from build123d import *

# Parameters (mm, degrees)
SALIENTE_EXTRUIR1_DEPTH      = 20
SALIENTE_EXTRUIR1_DEPTH_BACK = 15
CROQUIS1_R                   = 3.25
CROQUIS1_3_R                 = 7.5
CROQUIS1_3_R_2               = 3.25
SALIENTE_EXTRUIR2_DEPTH      = 3
SALIENTE_EXTRUIR3_DEPTH      = 2


with BuildPart() as part:
    # Croquis1 → Saliente-Extruir1 (new, two sides: drawn at the far end of the back side and taken through both)
    with BuildSketch(Plane(origin=(0, 0, 0), x_dir=(1, 0, 0), z_dir=(0, 1, 0)).offset(-SALIENTE_EXTRUIR1_DEPTH_BACK)):
        with Locations(Location((0, 0, 0), (0, 0, 270))):
            Circle(CROQUIS1_R)
    extrude(amount=SALIENTE_EXTRUIR1_DEPTH + SALIENTE_EXTRUIR1_DEPTH_BACK)

    # Croquis1_3 → Saliente-Extruir2 (add, symmetric)
    with BuildSketch(Plane(origin=(0, 0, 0), x_dir=(1, 0, 0), z_dir=(0, 1, 0))):
        with Locations(Location((0, 0, 0), (0, 0, 270))):
            Circle(CROQUIS1_3_R)
        with Locations(Location((0, 0, 0), (0, 0, 270))):
            Circle(CROQUIS1_3_R_2, mode=Mode.SUBTRACT)
    extrude(amount=SALIENTE_EXTRUIR2_DEPTH, both=True)

    # Croquis2 → Saliente-Extruir3 (add)
    with BuildSketch(Plane(origin=(0, 20, 0), x_dir=(1, 0, 0), z_dir=(0, 1, 0))):
        with BuildLine():
            Line((0, 3.25), (20, 3.25))
            ThreePointArc((20, 3.25), (23.25, 0), (20, -3.25))
            Line((20, -3.25), (0, -3.25))
            ThreePointArc((0, -3.25), (-3.25, 0), (0, 3.25))
        make_face()
    extrude(amount=SALIENTE_EXTRUIR3_DEPTH)


solid = part.part
Design review of the part built by this model. Coordinates are the model's own, in mm. A direction names the side the tool comes from. Give positions to 0.01 mm unless a question says otherwise; leave off trailing zeros. Loops run counter-clockwise (first coordinate to the right, second up) from the corner with the lowest first, then second, coordinate; pieces in that order, holes last. Notation, with made-up numbers: (32.5, 80) - (58.5, 80) arc R24 cw to (58.5, 115) - close; hole circle Ø5 at (-10.5, 18.5). An arc over 180 degrees is marked (long way). Use CSV: the item, a comma, the result in double quotes. Start each with the question number.
1. Add section B-B (x = 5.5). State the section outline as (y, z) points.
2. Add section A-A (z = 0). State the section outline as (x, y) points.
3. Add section D-D (x = 19). State the section outline as (y, z) points.
4. Add section C-C (y = -12). State the section outline as (x, z) points.
5. Insertion check: P1, Ø0.6, axis at x = 12.5, y = 21, coming from the -Z side; P2, Ø5, axis at y = -1, z = -3, coming from the -X side; P3, Ø1.5, axis at x = -0.5, y = -8.5, coming from the +Z side. Each pin has a flat end and moves straight along its axis. Give the tip position at first contact, or say it passes through.
6. Wall thickness on L1, parallel to Y at x = -3, z = 3.25; L2, parallel to X at y = -13, z = 0; L3, parallel to Z at x = 21, y = 20.5: over which ranges is each line inside the solid? List them lowest first.
7. Machinability: for faces 4 (the flat face through (-2, 3, 3)), 5 (the flat face through (-2, -3, 3)), 6 (the flat face through (10, 21, -3.25)), 7 (the flat face through (10, 21, 3.25)), which of the approach directions +Z, -Z, +X, -X, +Y, -Y give a long, thin tool a straight path to every point of the face, cutting with its end or side? Answer none if there is none.
8. Draft analysis for pull direction Y (two halves, no side actions). For faces 1 (the flat face through (0, -15, 0)), 2 (the cylindrical face through (23.25, 20.99, -0.07)), 3 (the cylindrical face through (-3.222, 12.367, -0.423)), state which applies: released by +Y, released by -Y, zero draft, split by the parting line, or undercut.
Results found:
1,outline,"(-3, -5.1) - (3, -5.1) - (3, 5.1) - (-3, 5.1) - close; (20, -3.25) - (22, -3.25) - (22, 3.25) - (20, 3.25) - close"
2,outline,"(-7.5, -3) - (-3.25, -3) - (-3.25, -15) - (3.25, -15) - (3.25, -3) - (7.5, -3) - (7.5, 3) - (3.25, 3) - (3.25, 20) - (23.25, 20) - (23.25, 22) - (-3.25, 22) - (-3.25, 3) - (-7.5, 3) - close"
3,outline,"(20, -3.25) - (22, -3.25) - (22, 3.25) - (20, 3.25) - close"
4,outline,"circle Ø6.5 at (0, 0)"
5,P1,"stops at z = -3.25"
5,P2,"stops at x = -7.48"
5,P3,"stops at z = 3.25"
6,L1,"y = -3 to 3"
6,L2,"x = -3.25 to 3.25"
6,L3,"z = -3.09 to 3.09"
7,face 4,"none"
7,face 5,"-Y"
7,face 6,"-Z, +X, -X, +Y"
7,face 7,"+Z, +X, -X, +Y"
8,face 1,"released by -Y"
8,face 2,"zero draft"
8,face 3,"undercut"
